CAD build for the part. Positions are in the model's coordinates, mm. Face numbers are marked on the shaded views. A direction names the side the tool comes from. Coordinates: 2 decimals unless noted, no trailing zeros. Order: outer loops, then holes, each group sorted by start corner. A loop starts at its lowest first (then second) coordinate and runs counter-clockwise, first axis right, second up. Notation, with made-up numbers: (21.5, -1.75) - (56.5, -1.75) arc R28 cw to (56.5, 24.25) - close; hole circle Ø9 at (32, -36). An arc over 180 degrees is marked (long way). Return JSON: item names as keys, results as strings.
Autodesk Inventor part; units mm, degrees
ref_plane "Start Plane" through (0, 0, 0) normal (0, 0, 1) x (1, 0, 0)
ref_plane "End Plane" through (0, 0, 270) normal (0, 0, 1) x (1, 0, 0)
ref_plane "YZ Plane" through (0, 0, 0) normal (1, 0, 0) x (0, 1, 0)
ref_plane "Start Plane" through (0, 0, 0) normal (0, 0, 1) x (1, 0, 0)
ref_plane "End Plane" through (0, 0, 270) normal (0, 0, 1) x (1, 0, 0)
sketch "Sketch" plane through (0, 0, 0) normal (0, 0, 1) x (1, 0, 0)
  line L0 (-50, -44) -> (-50, 44)
  line L1 (-44, 50) -> (44, 50)
  line L2 (50, 44) -> (50, -44)
  line L3 (44, -50) -> (-44, -50)
  arc A0 (-50, -44) -> (-44, -50) centre (-44, -44) ccw
  arc A1 (50, 44) -> (44, 50) centre (44, 44) ccw
  arc A2 (-44, 50) -> (-50, 44) centre (-44, 44) ccw
  arc A3 (44, -50) -> (50, -44) centre (44, -44) ccw
  arc A4 (-44, 47) -> (-47, 44) centre (-44, 44) ccw
  line L4 (-44, 47) -> (44, 47)
  arc A5 (47, 44) -> (44, 47) centre (44, 44) ccw
  line L5 (47, 44) -> (47, -44)
  arc A6 (44, -47) -> (47, -44) centre (44, -44) ccw
  line L6 (44, -47) -> (-44, -47)
  arc A7 (-47, -44) -> (-44, -47) centre (-44, -44) ccw
  line L7 (-47, -44) -> (-47, 44)
  line L8 (0, 71.7397) -> (0, -71.7397) construction
  line L9 (-71.7397, 0) -> (71.7397, 0) construction
  dimension "d7" = 6
  dimension "d9" = 100
  dimension "d11" = 100
  dimension "d12" = 3
  dimension "d15" = 50
  dimension "d16" = 50
extrude "Body" add sketch "Sketch" along normal up to surface (270 mm away) from surface at 0
sketch "Sketch3" plane through (0, 0, 0) normal (0, 0, 1) x (1, 0, 0)
  line L0 (0, 0) -> (10, 0)
ref_plane "Work Plane3" through (0, 0, 0) normal (0, -1, 0) x (1, 0, 0)
sketch "Sketch5" plane through (44, 50, 270) normal (0, 1, 0) x (1, 0, 0)
  point P0 (-44, 270)
sketch "Sketch6" plane through (-44, -50, 0) normal (0, -1, 0) x (1, 0, 0)
  line L0 (88, 0) -> (88, 270)
  line L1 (0, 0) -> (0, 270)
  line L2 (88, 0) -> (0, 0)
  line L3 (0, 0) -> (0, 141.42)
  line L4 (0, 141.42) -> (88, 141.42)
  line L5 (88, 141.42) -> (88, 0)
  line L6 (88, 4.24) -> (0, 4.24)
  line L7 (0, 4.24) -> (0, 137.24)
  line L8 (0, 137.24) -> (88, 137.24)
  line L9 (88, 137.24) -> (88, 4.24)
  line L10 (88, 146.42) -> (0, 146.42)
  line L11 (0, 146.42) -> (0, 216.42)
  line L12 (0, 216.42) -> (88, 216.42)
  line L13 (88, 216.42) -> (88, 146.42)
  point P0 (44, 0)
  point P1 (44, 141.42)
  point P2 (0, 146.42)
  point P3 (0, 4.24)
  dimension "d19" = 4.24
  dimension "d20" = 141.42
  dimension "d21" = 133
  dimension "d22" = 70
  dimension "d23" = 5
extrude "Extrusion2" cut sketch "Sketch6" against normal blind 3 contours L6 L1 L8 L0 | L10 L1 L12 L0
sketch "Sketch4" plane through (0, 0, 0) normal (0, -1, 0) x (1, 0, 0)
  line L0 (-2, 0) -> (12, 0)
  line L1 (-2, 270) -> (12, 270)
  dimension "d18" = 270
equation "\"d7\" = G_IR"
equation "\"d9\" = G_W"
equation "\"d11\" = G_H"
equation "\"d12\" = G_T"
equation "\"d15\" = 0.5 * d9"
equation "\"d16\" = 0.5 * d11"
equation "\"d3\" = G_L"
equation "\"G_W\" = 100"
equation "\"G_H\" = 100"
equation "\"G_T\" = 3"
equation "\"G_IR\" = 6"
equation "\"G_L\" = d18"
equation "\"G_OFFSET_START\" = 0"
equation "\"G_OFFSET_END\" = 0"
properties part number "ISO 10799-2 - 100x100x3 - 270" material "Steel, Mild"
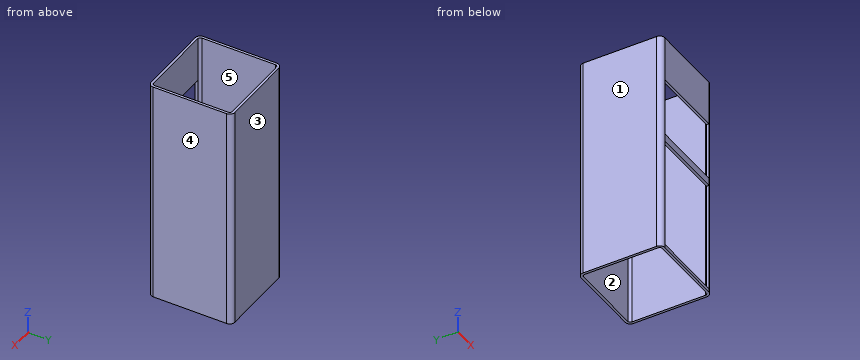
Item 1: Band-saw the part on D-D, the plane z = 90. List the corners of the cut face in (x, y), then the cut area to 3 significant figures.
Findings below:
{"outline": "(-50, -44) arc R6 ccw to (-44, -50) - (-44, -47) arc R3 cw to (-47, -44) - (-47, 44) arc R3 cw to (-44, 47) - (44, 47) arc R3 cw to (47, 44) - (47, -44) arc R3 cw to (44, -47) - (44, -50) arc R6 ccw to (50, -44) - (50, 44) arc R6 ccw to (44, 50) - (-44, 50) arc R6 ccw to (-50, 44) - close", "area": "877 mm²"}
Item 2: Band-saw the part on C-C, the plane x = 5. List the corners of the cut face in (y, z), then the cut area to 3 significant figures.
Findings below:
{"outline": "(-50, 0) - (-47, 0) - (-47, 4.24) - (-50, 4.24) - close; (-50, 137.24) - (-47, 137.24) - (-47, 146.42) - (-50, 146.42) - close; (-50, 216.42) - (-47, 216.42) - (-47, 270) - (-50, 270) - close; (47, 0) - (50, 0) - (50, 270) - (47, 270) - close", "area": "1,010 mm²"}
Item 3: Wall check: L1, parallel to X at y = 29, z = 246; L2, parallel to Y at x = -18, z = 162. Give the ranges that are in metal, low to high. Write a range as [from, to].
Findings below:
{"L1": "x = [-50, -47], [47, 50]", "L2": "y = [47, 50]"}
Item 4: Drop flat-ended pins along their axis: P1, Ø2.5, axis at y = -49, z = 197.5, coming from the +X side; P2, Ø0.9, axis at y = -48.5, z = 62, coming from the +X side; P3, Ø5, axis at x = -18.5, z = 184, coming from the -Y side. Give the stop position or say it passes through.
Findings below:
{"P1": "stops at x = 48.68", "P2": "stops at x = 48.43", "P3": "stops at y = 47"}
Item 5: Which spindle directions (+Z, -Z, +X, -X, +Y, -Y) get a long thin tool onto all of the face, cutting with end or side? Do the marked faces 4 and 5. Say none if no direction does.
Findings below:
{"face 4": "+Z, -Z, +X, +Y, -Y", "face 5": "+Z, -Z"}
Item 6: Band-saw the part on B-B, the plane z = 251.5. List the corners of the cut face in (x, y), then the cut area to 3 significant figures.
Findings below:
{"outline": "(-50, -44) arc R6 ccw to (-44, -50) - (44, -50) arc R6 ccw to (50, -44) - (50, 44) arc R6 ccw to (44, 50) - (-44, 50) arc R6 ccw to (-50, 44) - close; hole (-47, -44) arc R3 ccw to (-44, -47) - (44, -47) arc R3 ccw to (47, -44) - (47, 44) arc R3 ccw to (44, 47) - (-44, 47) arc R3 ccw to (-47, 44) - close", "area": "1,140 mm²"}
Item 7: Band-saw the part on A-A, the plane y = 38. List the corners of the cut face in (x, z).
Findings below:
{"outline": "(-50, 0) - (-47, 0) - (-47, 270) - (-50, 270) - close; (47, 0) - (50, 0) - (50, 270) - (47, 270) - close"}
Item 8: Mould opens along X. For the marked faces 1, 2 and 3 say: released by +X, released by -X, zero draft, split by the parting line, or undercut.
Findings below:
{"face 1": "released by -X", "face 2": "undercut", "face 3": "zero draft"}
